Build history of the part. All positions in model axes, mm. A direction names the side the tool comes from. Give positions to 0.01 mm unless a question says otherwise; leave off trailing zeros. Order: outer loops, then holes, each group sorted by start corner. A loop starts at its lowest first (then second) coordinate and runs counter-clockwise, first axis right, second up. Notation, with made-up numbers: M 27.5,46 L 66.5,46 A19 ccw 66.5,69 Z; hole C 13.25,77.5 d10. An arc over 180 degrees is marked long. One line per item, written item: value. Start each with the question number.
from build123d import *

# Parameters (mm, degrees)
SALIENTE_EXTRUIR1_DEPTH = 5
CORTAR_EXTRUIR1_DEPTH   = 1
CORTAR_EXTRUIR1_DRAFT   = -10
CROQUIS3_W              = 20
CROQUIS3_H              = 3.682271405
CORTAR_EXTRUIR3_DEPTH   = 13.68857754
CROQUIS4_R              = 2
SALIENTE_EXTRUIR2_DEPTH = 7.5


with BuildPart() as part:
    # Croquis1 → Saliente-Extruir1 (new body)
    with BuildSketch(Plane(origin=(0, 0, 0), x_dir=(1, 0, 0), z_dir=(0, 1, 0))):
        with BuildLine():
            Line((-3, -7), (-3, 7))
            ThreePointArc((-3, 7), (0, 10), (3, 7))
            Line((3, 7), (3, -7))
            ThreePointArc((3, -7), (0, -10), (-3, -7))
        make_face()
    extrude(amount=SALIENTE_EXTRUIR1_DEPTH)


with BuildPart() as cortar_extruir1_tool:
    # Croquis2 → Cortar-Extruir1 (with draft: the straight prism first)
    with BuildSketch(Plane(origin=(0, 5, 0), x_dir=(1, 0, 0), z_dir=(0, 1, 0))):
        with BuildLine():
            Line((-0.455587581, 6.404231625), (-0.455587581, 0.595768375))
            ThreePointArc((-0.455587581, 0.595768375), (-0.75, 0), (-0.455587581, -0.595768375))
            Line((-0.455587581, -0.595768375), (-0.455587581, -6.404231625))
            ThreePointArc((-0.455587581, -6.404231625), (0, -7.75), (0.455587581, -6.404231625))
            Line((0.455587581, -6.404231625), (0.455587581, -0.595768375))
            ThreePointArc((0.455587581, -0.595768375), (0.75, 0), (0.455587581, 0.595768375))
            Line((0.455587581, 0.595768375), (0.455587581, 6.404231625))
            ThreePointArc((0.455587581, 6.404231625), (0, 7.75), (-0.455587581, 6.404231625))
        make_face()
    extrude(amount=-CORTAR_EXTRUIR1_DEPTH)
    # Cortar-Extruir1: the draft: its side faces are tilted about the plane it starts from
    cortar_extruir1_sides = [cortar_extruir1_tool.faces().sort_by_distance(p)[0] for p in [
        (0, 4.5, -7.75),
        (-0.455587581, 4.5, -3.5),
        (-0.75, 4.5, 0),
        (-0.455587581, 4.5, 3.5),
        (0, 4.5, 7.75),
        (0.455587581, 4.5, 3.5),
        (0.75, 4.5, 0),
        (0.455587581, 4.5, -3.5),
    ]]
    draft(cortar_extruir1_sides, Plane(origin=(0, 5, 0), x_dir=(1, 0, 0), z_dir=(0, 1, 0)), CORTAR_EXTRUIR1_DRAFT)


with BuildPart() as part_1:
    add(part.part)

    # Cortar-Extruir1: cut by cortar_extruir1_tool
    add(cortar_extruir1_tool.part, mode=Mode.SUBTRACT)

    # Croquis3 → Cortar-Extruir3 (cut, through all)
    with BuildSketch(Plane(origin=(3, 0, 0), x_dir=(0, 0, -1), z_dir=(1, 0, 0))):
        with Locations((0, 2.458864298)):
            Rectangle(CROQUIS3_W, CROQUIS3_H)
    extrude(amount=-CORTAR_EXTRUIR3_DEPTH, mode=Mode.SUBTRACT)


with BuildPart() as cortar_extruir3_piece_1:
    # of the separate pieces the step leaves, piece 1, a body of its own (cortar_extruir3_pieces)
    add(part_1.part.solids().sort_by_distance((-3, 0, 7))[0])



with BuildPart() as cortar_extruir3_piece_2:
    # of the separate pieces the step leaves, piece 2, a body of its own (cortar_extruir3_pieces)
    add(part_1.part.solids().sort_by_distance((-3, 4.3, -7))[0])


with BuildPart() as cortar_extruir3_piece_1_1:
    add(cortar_extruir3_piece_1.part)

    add(cortar_extruir3_piece_2.part)  # Saliente-Extruir2 merges Cortar-Extruir3 piece 2
    # Croquis4 → Saliente-Extruir2 (add)
    with BuildSketch(Plane.XZ.offset(-4.3)):
        with Locations(Location((0, 0, 0), (0, 0, 80.440058332))):
            Circle(CROQUIS4_R)
    extrude(amount=SALIENTE_EXTRUIR2_DEPTH)


solid = cortar_extruir3_piece_1_1.part
1) Slice it at D-D (x = 1.75). List the corners of the cut face in (y, z).
2) Drill centre lines: line 1 (Y direction, x = -1.3, z = 2.5); line 2 (Y direction, x = 0.25, z = 0); line 3 (Z direction, x = 0.1, y = 4.25). Where is each one in solid material? Low to high.
3) Slice it at A-A (x = 0). List the corners of the cut face in (y, z).
4) Drop flat-ended pins along their axis: P1, Ø1.5, axis at x = -0.5, y = 2, coming from the -Z side; P2, Ø0.6, axis at x = 0, z = 0, coming from the +Y side. Give the stop position or say it passes through.
5) Pull direction Z, two halves, no side cores. Call faces 6 (the conical face through (0.024, 4.577, -7.675)), 7 (the cylindrical face through (-0.1, 4.6, -10)), 8 (the flat face through (0, 0, -2.4)): pulls with the +Z half, pulls with the -Z half, needs draft (parallel to the pull), parting line crosses it, or undercut.
6) Slice it at C-C (z = 8.5). List the corners of the cut face in (x, y).
7) Tool access for faces 1 (the cylindrical face through (1.9, 2.48, 0.62)), 2 (the flat face through (0, 4.3, 0)), 3 (the cylindrical face through (0.1, 4.6, 10)), 4 (the cylindrical face through (-0.1, 0.3, -10)), 5 (the cylindrical face through (1.9, -1.58, 0.62)): list every direction of +Z, -Z, +X, -X, +Y, -Y with a clear straight run to the whole face (end or side of a thin tool).
8) Slice it at B-B (z = 4.25). List the corners of the cut face in (x, y), plus the area to 3 significant figures.
Results list:
1. outline: M -3.2,-0.97 L 0,-0.97 L 0,-9.44 L 0.62,-9.44 L 0.62,-0.97 L 4.3,-0.97 L 4.3,-9.44 L 5,-9.44 L 5,9.44 L 4.3,9.44 L 4.3,0.97 L 0.62,0.97 L 0.62,9.44 L 0,9.44 L 0,0.97 L -3.2,0.97 Z
2. line 1: y = 0 to 0.62, 4.3 to 5
2. line 2: y = -3.2 to 4.3
2. line 3: z = -2 to 2
3. outline: M -3.2,-2 L 0,-2 L 0,-10 L 0.62,-10 L 0.62,-2 L 4.3,-2 L 4.3,2 L 0.62,2 L 0.62,10 L 0,10 L 0,2 L -3.2,2 Z; M 4.3,-10 L 5,-10 L 5,-7.75 L 4.3,-7.63 Z; M 4.3,7.63 L 5,7.75 L 5,10 L 4.3,10 Z
4. P1: stops at z = -2
4. P2: stops at y = 4.3
5. face 6: undercut
5. face 7: pulls with the -Z half
5. face 8: needs draft
6. outline: M -2.6,0 L 2.6,0 L 2.6,0.62 L -2.6,0.62 Z; M -2.6,4.3 L 2.6,4.3 L 2.6,5 L -2.6,5 Z
7. face 1: none
7. face 2: +Y
7. face 3: +Z, +Y, -Y
7. face 4: -Z, +Y, -Y
7. face 5: -Y
8. outline: M -3,0 L 3,0 L 3,0.62 L -3,0.62 Z; M -3,4.3 L -0.33,4.3 L -0.46,5 L -3,5 Z; M 0.33,4.3 L 3,4.3 L 3,5 L 0.46,5 Z
8. area: 7.35 mm²
